Autodesk Inventor part; units mm, degrees
ref_plane "YZ Plane" through (0, 0, 0) normal (1, 0, 0) x (0, 1, 0)
ref_plane "XZ Plane" through (0, 0, 0) normal (0, 1, 0) x (-1, 0, 0)
ref_plane "XY Plane" through (0, 0, 0) normal (0, 0, 1) x (1, 0, 0)
sketch "Sketch1" plane through (0, 0, 0) normal (0, 1, 0) x (-1, 0, 0)
  circle A0 centre (0, 0) radius 12.7
  circle A1 centre (0, 0) radius 3.302
  dimension "d0" = 25.4
  dimension "d1" = 6.604
extrude "Extrusion1" add sketch "Sketch1" along normal blind 12.7
sketch "Sketch2" plane through (0, 12.7, 0) normal (0, 1, 0) x (1, 0, 0)
  line L0 (0, 0) -> (0, -5.08)
  line L1 (0, -5.08) -> (0, 0)
  line L2 (0, 0) -> (0, 5.08)
  circle A0 centre (0, -5.08) radius 1.1049
  circle A1 centre (0, 5.08) radius 1.1049
  dimension "d4" = 5.08
  dimension "d5" = 5.08
  dimension "d6" = 2.2098
  dimension "d7" = 2.2098
extrude "Extrusion2" cut sketch "Sketch2" against normal blind 4.445
sketch "Sketch3" plane through (0, 0, 0) normal (0, -1, 0) x (1, 0, 0)
  line L0 (0, 0) -> (0, 5.08)
  line L1 (0, 5.08) -> (0, -5.08)
  circle A0 centre (0, 5.08) radius 1.1049
  circle A1 centre (0, -5.08) radius 1.1049
  dimension "d10" = 5.08
  dimension "d11" = 10.16
  dimension "d14" = 2.2098
  dimension "d15" = 2.2098
extrude "Extrusion3" cut sketch "Sketch3" against normal blind 1.905
properties part number "PolarisPost_HeightAdjustment_0p5in_smallholesfrom0p79to0p81"
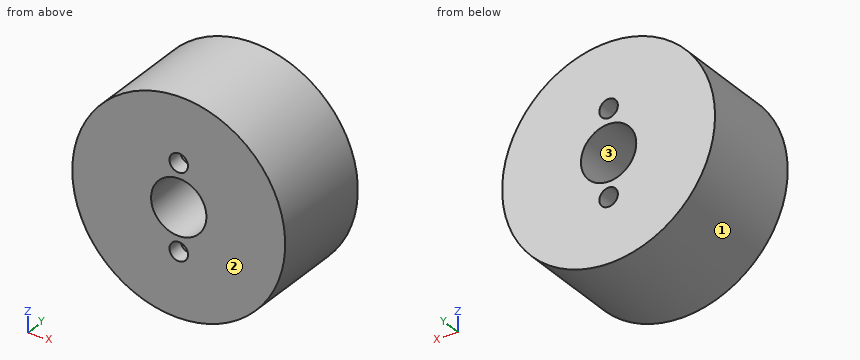
Read the model definition and answer for the solid it produces. Units are mm, in the model's axes. Face numbers are marked on the shaded views. Give positions to 0.01 mm unless a question says otherwise; leave off trailing zeros. Write each loop counter-clockwise with the first axis right and the second up, starting at its lowest first coordinate (ties: lowest second). Pieces come first, ordered by that corner, then holes. Notation, with made-up numbers: M 71.5,0.25 L 116.5,0.25 A24 ccw 116.5,25.25 Z; hole C -22,-30.5 d8. An arc over 180 degrees is marked long. One line per item, written item: value. Start each with the question number.
(1) Find section D-D (y = 6.5). Determine the outline of the cut face in (x, z), plus the area to 3 significant figures.
(2) Find section A-A (x = 0). Determine the outline of the cut face in (y, z) (3 decimals).
(3) Find section B-B (z = 0). Determine the outline of the cut face in (x, y).
(4) Determine the mould class of the marked faces 1, 2 and 3 for opening direction X: pulls with the +X half, pulls with the -X half, needs draft (parallel to the pull), parting line crosses it, or undercut.
(5) Find section C-C (z = 5.08). Determine the outline of the cut face in (x, y) (3 decimals).
(6) Find the intervals of material crossed by line 1 (Z direction, x = 0, y = 0.45); line 2 (Z direction, x = -1.25, y = 10); line 3 (Z direction, x = 2.5, y = 9.75), in increasing order.
(7) Flat-ended cylindrical pins translate along their axes: pin 1 Ø0.7 at (x, z) = (0.5, -5) entering from -Y (3 decimals); pin 2 Ø3 at (x, y) = (3.5, 3) entering from -Z; pin 3 Ø6 at (y, z) = (1.5, 4) entering from +X. Find the tip coordinate at first contact, or state that the pin passes through.
Results below:
1. outline: C 0,0 d25.4; hole C 0,0 d6.6
1. area: 472 mm^2
2. outline: M 0,-12.7 L 12.7,-12.7 L 12.7,-6.185 L 8.255,-6.185 L 8.255,-3.975 L 12.7,-3.975 L 12.7,-3.302 L 0,-3.302 L 0,-3.975 L 1.905,-3.975 L 1.905,-6.185 L 0,-6.185 Z; M 0,3.302 L 12.7,3.302 L 12.7,3.975 L 8.255,3.975 L 8.255,6.185 L 12.7,6.185 L 12.7,12.7 L 0,12.7 L 0,6.185 L 1.905,6.185 L 1.905,3.975 L 0,3.975 Z
3. outline: M -12.7,0 L -3.3,0 L -3.3,12.7 L -12.7,12.7 Z; M 3.3,0 L 12.7,0 L 12.7,12.7 L 3.3,12.7 Z
4. face 1: parting line crosses it
4. face 2: needs draft
4. face 3: undercut
5. outline: M -11.64,0 L -1.105,0 L -1.105,1.905 L 1.105,1.905 L 1.105,0 L 11.64,0 L 11.64,12.7 L 1.105,12.7 L 1.105,8.255 L -1.105,8.255 L -1.105,12.7 L -11.64,12.7 Z
6. line 1: z = -12.7 to -6.18, -3.98 to -3.3, 3.3 to 3.98, 6.18 to 12.7
6. line 2: z = -12.64 to -3.06, 3.06 to 12.64
6. line 3: z = -12.45 to -2.16, 2.16 to 12.45
7. pin 1: stops at y = 1.905
7. pin 2: stops at z = -12.54
7. pin 3: stops at x = 12.66
